Autodesk Inventor part; units mm, degrees
ref_plane "YZ Plane" through (0, 0, 0) normal (1, 0, 0) x (0, 1, 0)
ref_plane "XZ Plane" through (0, 0, 0) normal (0, 1, 0) x (-1, 0, 0)
ref_plane "XY Plane" through (0, 0, 0) normal (0, 0, 1) x (1, 0, 0)
sketch "Sketch1" plane through (0, 0, 0) normal (0, 0, 1) x (1, 0, 0)
  arc A0 (-21.2132, -1.5875) -> (-21.2132, 1.5875) centre (0, 0) ccw
  arc A1 (0, 33.9725) -> (-33.9725, 0) centre (0, 0) ccw
  line L0 (0, -33.9725) -> (-33.9725, -33.9725)
  line L1 (-33.9725, 0) -> (-33.9725, -33.9725)
  line L2 (0, 33.9725) -> (33.9725, 33.9725)
  line L3 (0, -33.9725) -> (33.9725, -33.9725)
  line L4 (33.9725, 0) -> (33.9725, -33.9725)
  line L5 (33.9725, 0) -> (33.9725, 33.9725)
  line L6 (0, 0) -> (-21.2655, 0) construction
  line L7 (-21.2132, 1.5875) -> (-22.8007, 1.5875)
  line L8 (-22.8007, 1.5875) -> (-22.8007, -1.5875)
  line L9 (-22.8007, -1.5875) -> (-21.2132, -1.5875)
  dimension "d0" = 42.545
  dimension "d1" = 67.945
  dimension "d29" = 1.5875
  dimension "d30" = 1.5875
  dimension "d31" = 1.5875
extrude "Extrusion1" add sketch "Sketch1" along normal mid plane 38.1
sketch "Sketch3" plane through (33.9725, -33.9725, 19.05) normal (1, 0, 0) x (0, 0, -1)
  line L0 (0, 67.945) -> (38.1, 67.945) construction
  line L1 (19.05, 67.945) -> (19.05, 0) construction
  line L2 (0, 0) -> (38.1, 0) construction
  point P0 (19.05, 33.9725)
  point P1 (19.05, 61.595)
  point P2 (19.05, 6.35)
  dimension "d13" = 6.35
  dimension "d14" = 6.35
split "Split1" plane through (0, 0, 0) removes the side toward (1, 0, 0)
sketch "Sketch4" plane through (0, 21.2725, -19.05) normal (1, 0, 0) x (0, 0, -1)
  point P0 (-19.05, -21.2725)
hole "Hole3" at (33.9725, 27.6225, 0) at (33.9725, -27.6225, 0) direction (-1, 0, 0) diameter 4.9784 depth 46.355 tip angle 118
sketch "Sketch5" plane through (-33.9725, -33.9725, 19.05) normal (-1, 0, 0) x (0, 0, 1)
  line L0 (0, 0) -> (-38.1, 0) construction
  line L1 (-31.75, 0) -> (-31.75, 33.9725) construction
  line L2 (-6.35, 0) -> (-6.35, 33.9725) construction
  line L3 (0, 33.9725) -> (-38.1, 33.9725) construction
  line L4 (-38.1, 0) -> (-38.1, 33.9725) construction
  line L5 (0, 33.9725) -> (0, 0) construction
  line L6 (-19.05, 33.9725) -> (-19.05, 0) construction
  point P0 (-31.75, 10.16)
  point P1 (-6.35, 10.16)
  point P2 (-19.05, 10.16)
  dimension "d32" = 6.35
  dimension "d33" = 6.35
  dimension "d34" = 10.16
  dimension "d35" = 10.16
sketch "Sketch6" plane through (0, -33.9725, 19.05) normal (1, 0, 0) x (0, 0, -1)
  line L0 (0, 67.945) -> (38.1, 67.945) construction
  line L1 (6.35, 67.945) -> (6.35, 0) construction
  line L2 (0, 0) -> (38.1, 0) construction
  line L3 (31.75, 67.945) -> (31.75, 0) construction
  line L4 (0, 0) -> (0, 12.7) construction
  line L5 (38.1, 12.7) -> (38.1, 0) construction
  point P0 (19.05, 33.9725)
  point P1 (6.35, 6.35)
  point P2 (6.35, 61.595)
  point P3 (31.75, 61.595)
  point P4 (31.75, 6.35)
  dimension "d36" = 6.35
  dimension "d37" = 6.35
  dimension "d38" = 6.35
  dimension "d39" = 6.35
hole "Hole4" at (-33.9725, -23.8125, -12.7) at (-33.9725, -23.8125, 0) at (-33.9725, -23.8125, 12.7) direction (1, 0, 0) diameter 4.9784 depth 25.4 tip angle 118
hole "Hole5" at (0, 27.6225, 12.7) at (0, 27.6225, -12.7) at (0, -27.6225, -12.7) at (0, -27.6225, 12.7) direction (-1, 0, 0) diameter 4.9784 depth 9.525 tip angle 118
equation "\"d0\" = pipeDiameter"
equation "\"d1\" = pipeDiameter + 2 * outerRadius"
equation "\"d2\" = width"
equation "\"pipeDiameter\" = 42.545"
equation "\"outerRadius\" = 12.7"
equation "\"width\" = 38.1"
properties part number "gripperBracketA" material "Aluminum 6061"
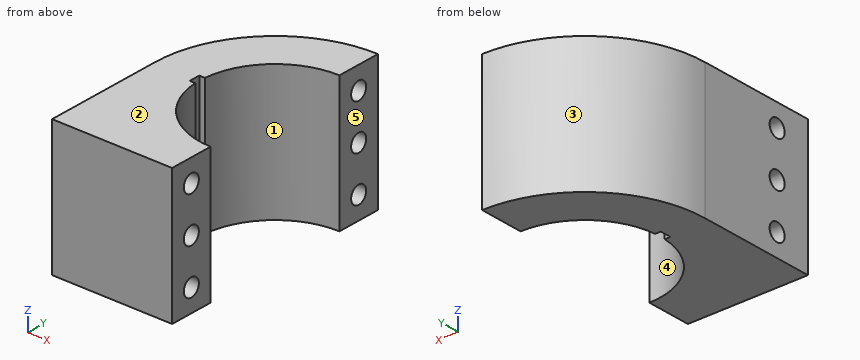
Check sheet for the modelled part. Datum: model origin and axes. Units: mm. Face numbers are marked on the shaded views. A direction names the side the tool comes from. Round coordinates to 2 decimals unless told otherwise and drop trailing zeros. Write each loop counter-clockwise with the first axis right and the second up, starting at its lowest first coordinate (ties: lowest second). Pieces come first, ordered by that corner, then holes. Notation, with made-up numbers: M 9,20 L 13,20 A4 cw 13,24 Z; hole C 13.5,40.5 d9. An arc over 180 degrees is marked long. Write item = value, one per line. Start each with the question number.
1. Release check for a two-part mould opening along Y. For the marked faces 1, 2 and 3 record: pulls with the +Y half, pulls with the -Y half, needs draft (parallel to the pull), parting line crosses it, or undercut.
2. Gauge pin test, flat ends, axial feed: pin 1 (4 mm diameter, centred on y = -23.81, z = -12.7, fed in from -X); pin 2 (8 mm diameter, centred on y = 27.62, z = 0, fed in from -X); pin 3 (3 mm diameter, centred on x = -16.5, z = -8.5, fed in from +Y). Record the tip position at first contact, or that the pin passes through.
3. Section check D-D, the plane y = -8. Record the cut outline in (x, z), then the cut area to 3 significant figures.
4. Scan lines: line 1 (Y direction, x = -3.5, z = -12.7); line 2 (Y direction, x = -3.75, z = 12.7); line 3 (Y direction, x = -11, z = 12). Record each from-to range of solid material in increasing order. Write a range as [from, to].
5. Section check C-C, the plane x = -23.5. Record the cut outline in (y, z).
6. Section check B-B, the plane x = -3. Record the cut outline in (y, z).
7. Tool access check on the marked faces 4 and 5. Record the directions out of +Z, -Z, +X, -X, +Y, -Y that give a thin tool (end or side, any length) a straight path to the whole face; none if there is none.
8. Section check A-A, the plane x = -19.5. Record the cut outline in (y, z).
Results found:
q1.face_1 = undercut
q1.face_2 = needs draft
q1.face_3 = pulls with the +Y half
q2.pin_1 = -8.28
q2.pin_2 = -24.42
q2.pin_3 = 30.48
q3.outline = M -33.97,-19.05 L -19.71,-19.05 L -19.71,19.05 L -33.97,19.05 Z
q3.area = 543 mm^2
q4.line_1 = [-33.97, -30.11], [-25.13, -20.98], [20.98, 25.13], [30.11, 33.79]
q4.line_2 = [-33.97, -30.11], [-25.13, -20.94], [20.94, 25.13], [30.11, 33.76]
q4.line_3 = [-33.97, -26.2], [-21.42, -18.21], [18.21, 32.14]
q5.outline = M -33.97,-19.05 L 24.53,-19.05 L 24.53,19.05 L -33.97,19.05 Z; hole C -23.81,-12.7 d4.98; hole C -23.81,0 d4.98; hole C -23.81,12.7 d4.98
q6.outline = M -33.97,-19.05 L -21.06,-19.05 L -21.06,19.05 L -33.97,19.05 Z; M 21.06,-19.05 L 33.84,-19.05 L 33.84,19.05 L 21.06,19.05 Z; hole C -27.62,-12.7 d4.98; hole C -27.62,0 d4.98; hole C -27.62,12.7 d4.98; hole C 27.62,-12.7 d4.98; hole C 27.62,0 d4.98; hole C 27.62,12.7 d4.98
q7.face_4 = +Z, -Z, +X
q7.face_5 = +Z, -Z, +X, +Y, -Y
q8.outline = M -33.97,-19.05 L -8.5,-19.05 L -8.5,19.05 L -33.97,19.05 Z; M 8.5,-19.05 L 27.82,-19.05 L 27.82,19.05 L 8.5,19.05 Z; hole C -23.81,-12.7 d4.98; hole C -23.81,0 d4.98; hole C -23.81,12.7 d4.98
